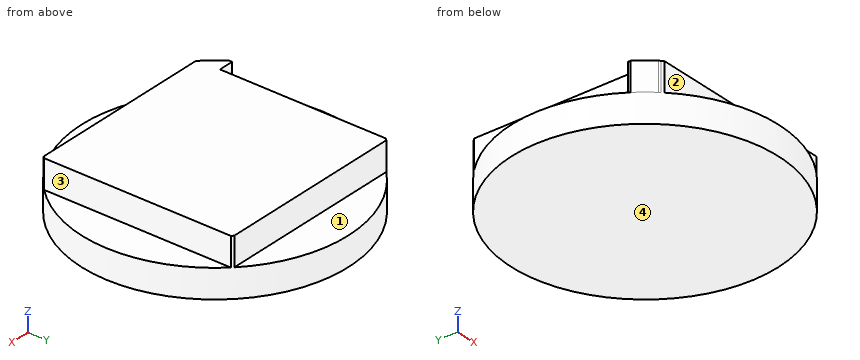
Autodesk Inventor part; units mm, degrees
ref_plane "YZ Plane" through (0, 0, 0) normal (1, 0, 0) x (0, 1, 0)
ref_plane "XZ Plane" through (0, 0, 0) normal (0, 1, 0) x (-1, 0, 0)
ref_plane "XY Plane" through (0, 0, 0) normal (0, 0, 1) x (1, 0, 0)
sketch "Skizze1" plane through (0, 0, 0) normal (0, 0, 1) x (1, 0, 0)
  circle A0 centre (0, 0) radius 7
  line L0 (-5, 5) -> (5, 5) construction
  line L1 (5, 5) -> (5, -5) construction
  line L2 (5, -5) -> (-5, -5) construction
  line L3 (-5, -5) -> (-5, 5) construction
  line L4 (-5, 5) -> (5, -5) construction
  line L5 (5, 5) -> (-5, -5) construction
  dimension "d0" = 14
  dimension "d1" = 10
  dimension "d2" = 10
extrude "Extrusion1" add sketch "Skizze1" along normal blind 1.5
sketch "Skizze4" plane through (0, 0, 1.5) normal (0, 0, 1) x (1, 0, 0)
  circle A0 centre (0, 0) radius 7 construction
  line L0 (-5, -5) -> (5, -5)
  line L1 (5, -5) -> (5, 5)
  line L2 (5, 5) -> (-5, 5)
  line L3 (-5, 5) -> (-5, -5)
  line L4 (-5, -5) -> (5, 5) construction
  line L5 (5, -5) -> (-5, 5) construction
  dimension "d9" = 10
  dimension "d10" = 10
extrude "Extrusion3" add sketch "Skizze4" along normal blind 1.5
sketch "Skizze5" plane through (0, 0, 3) normal (0, 0, 1) x (1, 0, 0)
  circle A0 centre (0, 0) radius 7
  circle A1 centre (0, 0) radius 7.3678
extrude "Extrusion4" cut sketch "Skizze5" against normal through all
sketch "Skizze6" plane through (0, 0, 1.5) normal (0, 0, 1) x (1, 0, 0)
  arc A0 (-5.7802, -3.9484) -> (-5, -4.899) centre (0, 0) ccw
  line L0 (-5, 4.899) -> (-5, -4.899)
  line L1 (-5, -3.8099) -> (-5.7802, -3.8099)
  line L2 (-5.7802, -3.8099) -> (-5.7802, -3.9484)
  line L3 (-5.0692, -4.8273) -> (-5, -4.8273)
  line L4 (-5, -4.8273) -> (-5, -3.8099)
extrude "Extrusion5" add sketch "Skizze6" along normal up to surface (1.5 mm away) contours L2 L1 L0 L3 A0
sketch "Skizze7" plane through (0, 0, 3) normal (0, 0, 1) x (1, 0, 0)
  arc A0 (-5.0692, -4.8273) -> (-5, -4.899) centre (0, 0) ccw
  line L0 (-5, -4.8273) -> (-5, -4.899)
  line L1 (-5, -4.8273) -> (-5.0692, -4.8273)
extrude "Extrusion6" add sketch "Skizze7" against normal up to surface (1.5 mm away)
properties part number "aruco_chip"
Could you check a few things on this model? Use its own coordinates, in mm. Face numbers are marked on the shaded views. A direction names the side the tool comes from. Give positions to 0.01 mm unless a question says otherwise; leave off trailing zeros. Write each loop counter-clockwise with the first axis right and the second up, starting at its lowest first coordinate (ties: lowest second). Pieces come first, ordered by that corner, then holes. Notation, with made-up numbers: (14.25, 75.5) -> (58.25, 75.5) arc R6 ccw to (58.25, 85.5) -> close; hole circle Ø4 at (62.5, -0.75). An arc over 180 degrees is marked (long way). Answer as CSV lines item,"result". Start each with the question number.
(1) If we section it at D-D, the plane z = 0.4: Write out the boundary of the cut face in (x, y), and give its area (3 significant figures).
(2) I'm going to push flat-ended pins straight in: pin 1 Ø1.6 at (x, y) = (0, -6) entering from +Z; pin 2 Ø0.6 at (x, z) = (-5, 2.5) entering from +Y; pin 3 Ø1.5 at (x, z) = (-5, 1) entering from -Y; pin 4 Ø2 at (x, y) = (-2, 4) entering from -Z. Where does each tip first touch, or does it pass through?
(3) Which directions (+Z, -Z, +X, -X, +Y, -Y) give clear straight access to the entire face, cutting with the end or side of a thin tool? Please do the marked faces 1, 2, 3 and 4.
(4) If we section it at B-B, the plane z = 1.85: Write out the boundary of the cut face in (x, y), and give its area (3 significant figures).
(5) Please list where these lines run through material, in increasing order: line 1 (X direction, y = 2.5, z = 1.75); line 2 (Z direction, x = -0.5, y = -5.75).
(6) If we section it at A-A, the plane x = 0: Write out the boundary of the cut face in (y, z), and give its area (3 significant figures).
Answer list:
1,outline,"circle Ø14 at (0, 0)"
1,area,"154 mm^2"
2,pin 1,"z = 1.5"
2,pin 2,"y = 5"
2,pin 3,"y = -5.56"
2,pin 4,"z = 0"
3,face 1,"+Z, +X, -X, +Y"
3,face 2,"+Z, +X, -X, -Y"
3,face 3,"+Z, +X, +Y, -Y"
3,face 4,"-Z, +X, -X, +Y, -Y"
4,outline,"(-5.78, -3.95) arc R7 ccw to (-5.07, -4.83) arc R7.94 ccw to (-5, -4.9) arc R7 ccw to (-4.9, -5) -> (4.9, -5) arc R7 ccw to (5, -4.9) -> (5, 4.9) arc R7 ccw to (4.9, 5) -> (-4.9, 5) arc R7 ccw to (-5, 4.9) -> (-5, -3.81) -> (-5.78, -3.81) -> close"
4,area,"100 mm^2"
5,line 1,"-5 to 5"
5,line 2,"0 to 1.5"
6,outline,"(-7, 0) -> (7, 0) -> (7, 1.5) -> (5, 1.5) -> (5, 3) -> (-5, 3) -> (-5, 1.5) -> (-7, 1.5) -> close"
6,area,"36.0 mm^2"
